Geometry: final body of the model. Coordinates: model frame, mm. Face numbers are marked on the shaded views. A direction names the side the tool comes from. Give positions to 0.01 mm unless a question says otherwise; leave off trailing zeros. Loops run counter-clockwise (first coordinate to the right, second up) from the corner with the lowest first, then second, coordinate; pieces in that order, holes last.
1. Section B-B, the plane z = 4.5. Output: boundary loops of the cut face in (x, y).
2. Draft query along Y for the marked faces 1, 2, 3 and 4. Return one class per face: +Y half, -Y half, draft (parallel to the pull), parting line (faces both ways), or undercut.
3. Access query for the marked faces 5, 6 and 7. Directions: +Z, -Z, +X, -X, +Y, -Y. A direction counts if a zero-diameter tool reaches every point of the face in a straight line with its end or side. Return the directions, or none.
4. First-contact query: P1, Ø3, axis at x = -8, z = 4, coming from the +Y side; P2, Ø3.5, axis at x = -5.5, y = -5, coming from the -Z side; P3, Ø6, axis at y = 5.5, z = 7.5, coming from the -X side; P4, Ø2, axis at y = 0.5, z = 1, coming from the +X side. Flat tips, straight axial feed; report the tip coordinate or a pass-through.
5. Material intervals for line 1 along Y through (x, z) = (-5.75, 0.5); line 2 along Z through (x, y) = (-8, -0.75); line 3 along Y through (x, z) = (-3, 8), sorted ascending.
6. Section A-A, the plane y = 0. Output: boundary loops of the cut face in (x, z).
7. Section C-C, the plane x = -6.75. State how many separate pieces and enclosed holes the cut face has, then the cut area to 3 significant figures.
from build123d import *

# Parameters (mm, degrees)
EXTRUDE_1_DEPTH          = 1
EXTRUDE_2_DEPTH          = 10
SKETCH_3_R               = 0.75
CUT_EXTRUDE_1_DEPTH      = 10
PATTERN_CIRCULAR_1_COUNT = 18
FILLET_1_R               = 1


with BuildPart() as part:
    # Эскиз1 → Бобышка-Вытянуть1 (new body)
    with BuildSketch(Plane.XY):
        with BuildLine():
            Line((0, 3.5), (-8.291561976, 3.5))
            ThreePointArc((-8.291561976, 3.5), (-9, 0), (-8.291561976, -3.5))
            Line((-8.291561976, -3.5), (0, -3.5))
            ThreePointArc((0, -3.5), (-3.5, 0), (0, 3.5))
        make_face()
    extrude(amount=EXTRUDE_1_DEPTH)

    # Эскиз2 → Бобышка-Вытянуть2 (add)
    with BuildSketch(Plane.XY.offset(1)):
        with BuildLine():
            Line((5.61e-07, 8), (-4.123105626, 8))
            ThreePointArc((-4.123105626, 8), (-9, 0), (-4.123105626, -8))
            Line((-4.123105626, -8), (2.99e-07, -8))
            ThreePointArc((2.99e-07, -8), (-8, 1.31e-07), (5.61e-07, 8))
        make_face()
    extrude(amount=EXTRUDE_2_DEPTH)

    # Эскиз3 → Вырез-Вытянуть1 (cut)
    with BuildSketch(Plane(origin=(0, 0, 0), x_dir=(1, 0, 0), z_dir=(0, 1, 0))):
        with Locations((0, -10)):
            Circle(SKETCH_3_R)
    cut_extrude_1 = extrude(amount=-CUT_EXTRUDE_1_DEPTH, mode=Mode.SUBTRACT)

    # Круговой массив1: Вырез-Вытянуть1 ×18 about axis
    pattern_circular_1_axis = Axis((0, 0, 0), (0, 0, -1))
    for i in range(1, PATTERN_CIRCULAR_1_COUNT):
        add(cut_extrude_1.rotate(pattern_circular_1_axis, i * 360 / PATTERN_CIRCULAR_1_COUNT), mode=Mode.SUBTRACT)

    # Скругление1
    fillet_1_edges = [part.edges().sort_by_distance(p)[0] for p in [
        (-8, 0, 1),
    ]]
    fillet(fillet_1_edges, radius=FILLET_1_R)


solid = part.part
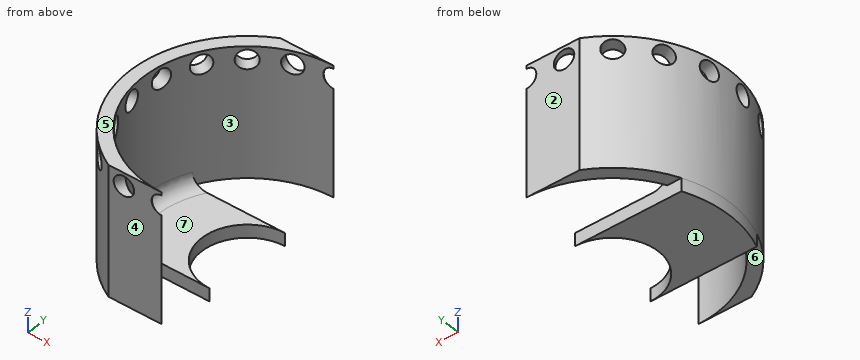
Answers below:
1. outline: (-4.12, -8) - (0, -8) arc R8 cw to (0, 8) - (-4.12, 8) arc R9 ccw to start
2. face 1: draft
2. face 2: +Y half
2. face 3: undercut
2. face 4: -Y half
3. face 5: +Z, +X, -X, +Y, -Y
3. face 6: -Z, +X, -X, -Y
3. face 7: +Z, +X
4. P1: stops at y = 6.22
4. P2: stops at z = 0
4. P3: stops at x = -8.65
4. P4: stops at x = -3.16
5. line 1: y = -3.5 to 3.5
5. line 2: z = 0 to 9.63, 10.37 to 11
5. line 3: y = -8 to -7.42, 7.42 to 8
6. outline: (-9, 0) - (-3.5, 0) - (-3.5, 1) - (-7, 1) arc R1 cw to (-8, 2) - (-8, 11) - (-9, 11) - close
7. separate pieces: 3
7. enclosed holes: 0
7. area: 39.5 mm2
